Input: part model. Units: mm. Frame: model coordinates. Face numbers are marked on the shaded views. A direction names the side the tool comes from. Coordinates: 2 decimals unless noted, no trailing zeros. Loops run counter-clockwise (first coordinate to the right, second up) from the corner with the lowest first, then second, coordinate; pieces in that order, holes last. Notation, with made-up numbers: M -38.5,-27 L -17.5,-27 A22 ccw -17.5,-13 Z; hole C 87.25,50 d1. An arc over 180 degrees is marked long. Use a Markdown table: item, result. Add a question column.
1. Draft query along Y for the marked faces 3, 4, 5 and 6. Return one class per face: +Y half, -Y half, draft (parallel to the pull), parting line (faces both ways), or undercut.
2. Section D-D on x = -379. Output: boundary loops of the cut face in (y, z) (3 decimals).
3. Pin query (flat end, axial travel): pin 1 (8 mm diameter, centred on y = 20, z = 8, fed in from -X); pin 2 (3 mm diameter, centred on x = -47.5, z = 8, fed in from -Y); pin 3 (6 mm diameter, centred on x = -64, y = -14, fed in from +Z). Return the tip coordinate at first contact, or that it passes through.
4. Section A-A on y = 0. Output: boundary loops of the cut face in (x, z) (3 decimals), then the cut area to 3 significant figures.
5. Line query: L1, parallel to Y at x = -120, z = -6 (3 decimals); L2, parallel to Z at x = -298, y = 19. Output: solid intervals per line, ascending. Write a range as [from, to].
6. Set-up query: the marked faces 1 and 2. Return all of +Z, -Z, +X, -X, +Y, -Y with unobstructed straight access to the full face (end or side cutting, diameter ignored); none if empty.
7. Section B-B on z = 2. Output: boundary loops of the cut face in (x, y) (3 decimals).
8. Section C-C on x = -171. Output: boundary loops of the cut face in (y, z) (3 decimals).
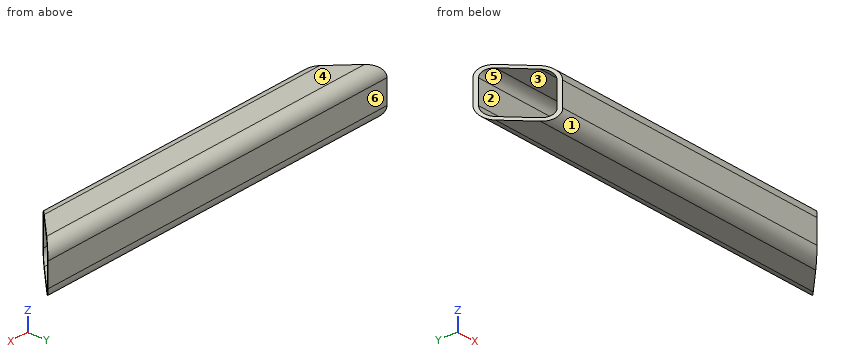
```python
from build123d import *

# Parameters (mm, degrees)
STRUCTURAL_MEMBER1_DEPTH = 406.4
CUT_EXTRUDE1_DEPTH       = 411.349558304


with BuildPart() as part:
    # Sketch11 → Structural Member1 (new body)
    with BuildSketch(Plane.ZY):
        with BuildLine():
            Line((-12.7, -25.4), (12.7, -25.4))
            ThreePointArc((12.7, -25.4), (21.680256121, -21.680256121), (25.4, -12.7))
            Line((25.4, -12.7), (25.4, 12.7))
            ThreePointArc((25.4, 12.7), (21.680256121, 21.680256121), (12.7, 25.4))
            Line((12.7, 25.4), (-12.7, 25.4))
            ThreePointArc((-12.7, 25.4), (-21.680256121, 21.680256121), (-25.4, 12.7))
            Line((-25.4, 12.7), (-25.4, -12.7))
            ThreePointArc((-25.4, -12.7), (-21.680256121, -21.680256121), (-12.7, -25.4))
        make_face()
        with BuildLine():
            Line((-12.7, -22.225), (12.7, -22.225))
            ThreePointArc((12.7, -22.225), (19.435192091, -19.435192091), (22.225, -12.7))
            Line((22.225, -12.7), (22.225, 12.7))
            ThreePointArc((22.225, 12.7), (19.435192091, 19.435192091), (12.7, 22.225))
            Line((12.7, 22.225), (-12.7, 22.225))
            ThreePointArc((-12.7, 22.225), (-19.435192091, 19.435192091), (-22.225, 12.7))
            Line((-22.225, 12.7), (-22.225, -12.7))
            ThreePointArc((-22.225, -12.7), (-19.435192091, -19.435192091), (-12.7, -22.225))
        make_face(mode=Mode.SUBTRACT)
    extrude(amount=STRUCTURAL_MEMBER1_DEPTH)

    # Sketch2 → Cut-Extrude1 (cut, through all)
    with BuildSketch(Plane.XY.offset(25.4)):
        Polygon((-406.4, 25.4), (-355.6, -25.4), (-406.4, -25.4), align=None)
        Polygon((0, 25.4), (-50.8, -25.4), (0, -25.4), align=None)
    extrude(amount=-CUT_EXTRUDE1_DEPTH, mode=Mode.SUBTRACT)


solid = part.part
```
Answers below:
| question | item | result |
|---|---|---|
| 1 | face 3 | undercut |
| 1 | face 4 | draft |
| 1 | face 5 | undercut |
| 1 | face 6 | +Y half |
| 2 | outline | M -2,-25.4 L 12.7,-25.4 A12.7 ccw 25.4,-12.7 L 25.4,12.7 A12.7 ccw 12.7,25.4 L -2,25.4 L -2,22.225 L 12.7,22.225 A9.525 cw 22.225,12.7 L 22.225,-12.7 A9.525 cw 12.7,-22.225 L -2,-22.225 Z |
| 3 | pin 1 | stops at x = -405 |
| 3 | pin 2 | stops at y = -23.6 |
| 3 | pin 3 | stops at z = 25.4 |
| 4 | outline | M -381,-25.4 L -25.4,-25.4 L -25.4,-22.225 L -381,-22.225 Z; M -381,22.225 L -25.4,22.225 L -25.4,25.4 L -381,25.4 Z |
| 4 | area | 2,260 mm² |
| 5 | L1 | y = [-25.4, -22.225], [22.225, 25.4] |
| 5 | L2 | z = [-23.73, -19.84], [19.84, 23.73] |
| 6 | face 1 | -Z, +X, -X, -Y |
| 6 | face 2 | +X, -X |
| 7 | outline | M -406.4,25.4 L -403.225,22.225 L -3.175,22.225 L 0,25.4 Z; M -358.775,-22.225 L -355.6,-25.4 L -50.8,-25.4 L -47.625,-22.225 Z |
| 8 | outline | M -25.4,-12.7 A12.7 ccw -12.7,-25.4 L 12.7,-25.4 A12.7 ccw 25.4,-12.7 L 25.4,12.7 A12.7 ccw 12.7,25.4 L -12.7,25.4 A12.7 ccw -25.4,12.7 Z; hole M -22.225,-12.7 A9.525 ccw -12.7,-22.225 L 12.7,-22.225 A9.525 ccw 22.225,-12.7 L 22.225,12.7 A9.525 ccw 12.7,22.225 L -12.7,22.225 A9.525 ccw -22.225,12.7 Z |
